Read the model definition and answer for the solid it produces. Units are mm, in the model's axes. Face numbers are marked on the shaded views. Give positions to 0.01 mm unless a question says otherwise; leave off trailing zeros. Write each loop counter-clockwise with the first axis right and the second up, starting at its lowest first coordinate (ties: lowest second). Pieces come first, ordered by that corner, then holes. Notation, with made-up numbers: M 22.25,-1 L 57.25,-1 A30 ccw 57.25,23 Z; hole C 33.25,35 d6. An arc over 180 degrees is marked long. Use a Markdown table: item, result. Add a question column.
Item 1: A cutting plane is placed at A-A on x = 55.5. Determine the outline of the cut face in (y, z), then the cut area to 3 significant figures.
Item 2: Given P1, Ø10, axis at x = 97.5, y = -38.5, coming from the +Z side; P2, Ø3, axis at x = 80.5, z = -8, coming from the +Y side; P3, Ø3, axis at x = 27, z = -3.5, coming from the -Y side; P4, Ø4, axis at y = -60, z = -7.5, coming from the +X side, each flat-ended and moving along its own axis, determine where each tip first touches the part or whether it passes through.
Item 3: A cutting plane is placed at C-C on z = -8. Count the separate pieces of the cut face and the enclosed holes in it, then the cut area to 3 significant figures.
Item 4: Consider probe 1 along Y at (x, z) = (114, -10.5); probe 2 along X at (y, z) = (-56.5, -9.25); probe 3 along X at (y, z) = (27.5, -4.75). Determine where each line is inside the solid, lowest interval first. Write a range as [from, to].
Item 5: A cutting plane is placed at B-B on y = -19. Determine the outline of the cut face in (x, z), then the cut area to 3 significant figures.
Item 6: The mould has two halves that part along Y. Classify the marked faces 1 and 2: pulls with the +Y half, pulls with the -Y half, needs draft (parallel to the pull), parting line crosses it, or undercut.
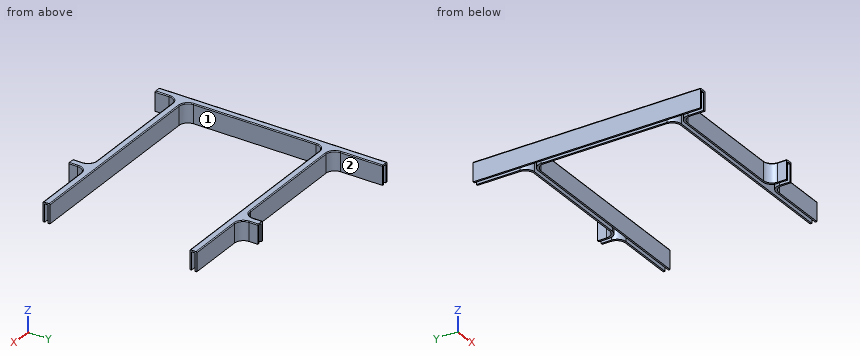
from build123d import *

# Parameters (mm, degrees)
F0_W     = 2
F0_H     = 10
F0_H_2   = 1
F1_DEPTH = 0.9
F0_W_2   = 1
F0_H_3   = 130
F0_W_3   = 76
F0_W_4   = 38
F2_DEPTH = 11
F3_R     = 5
F4_R     = 0.5


with BuildPart() as f1:
    # F0 (on Top) → F1 (new body)
    with BuildSketch(Plane.XY):
        Polygon((-1, -65), (1, -65), (1, -51), (1, -49), (1, 33), (1, 35), (1, 65), (-1, 65), align=None)
        Polygon((1, 35), (1, 33), (2, 33), (79, 33), (81, 33), (120, 33), (120, 35), (82, 35), (81, 35), (79, 35), (78, 35), (2, 35), align=None)
        with Locations((80, 41)):
            Rectangle(F0_W, F0_H)
        with Locations((80, 35.5)):
            Rectangle(F0_W, F0_H_2)
        Polygon((1, -49), (1, -51), (2, -51), (78, -51), (79, -51), (81, -51), (82, -51), (120, -51), (120, -49), (81, -49), (79, -49), (2, -49), align=None)
        with Locations((80, -57)):
            Rectangle(F0_W, F0_H)
        with Locations((80, -51.5)):
            Rectangle(F0_W, F0_H_2)
    extrude(amount=-F1_DEPTH)

    # F0 (on Top) → F2 (join)
    with BuildSketch(Plane.XY):
        Polygon((1, -51), (1, -65), (2, -65), (2, -52), (2, -51), align=None)
        with Locations((-1.5, 0)):
            Rectangle(F0_W_2, F0_H_3)
        Polygon((1, 33), (1, -49), (2, -49), (2, -48), (2, 32), (2, 33), align=None)
        with Locations((40, -51.5)):
            Rectangle(F0_W_3, F0_H_2)
        Polygon((2, 65), (1, 65), (1, 35), (2, 35), (2, 36), align=None)
        Polygon((2, -48), (2, -49), (79, -49), (79, -48), (78, -48), align=None)
        with Locations((78.5, -51.5)):
            Rectangle(F0_W_2, F0_H_2)
        with Locations((78.5, -57)):
            Rectangle(F0_W_2, F0_H)
        Polygon((79, 33), (2, 33), (2, 32), (78, 32), (79, 32), align=None)
        with Locations((80, -48.5)):
            Rectangle(F0_W, F0_H_2)
        with Locations((40, 35.5)):
            Rectangle(F0_W_3, F0_H_2)
        with Locations((80, 32.5)):
            Rectangle(F0_W, F0_H_2)
        Polygon((81, -48), (81, -49), (120, -49), (120, -48), (82, -48), align=None)
        with Locations((81.5, -51.5)):
            Rectangle(F0_W_2, F0_H_2)
        with Locations((81.5, -57)):
            Rectangle(F0_W_2, F0_H)
        with Locations((78.5, 35.5)):
            Rectangle(F0_W_2, F0_H_2)
        with Locations((78.5, 41)):
            Rectangle(F0_W_2, F0_H)
        Polygon((120, 33), (81, 33), (81, 32), (82, 32), (120, 32), align=None)
        with Locations((101, -51.5)):
            Rectangle(F0_W_4, F0_H_2)
        with Locations((81.5, 35.5)):
            Rectangle(F0_W_2, F0_H_2)
        with Locations((81.5, 41)):
            Rectangle(F0_W_2, F0_H)
        with Locations((101, 35.5)):
            Rectangle(F0_W_4, F0_H_2)
    extrude(amount=-F2_DEPTH)

    # F3
    f3_edges = [f1.edges().sort_by_distance(p)[0] for p in [
        (78, -52, -5.5),
        (81, -51, -5.95),
        (82, -52, -5.5),
        (79, -51, -5.95),
        (1, -49, -5.95),
        (1, -51, -5.95),
        (2, -52, -5.5),
        (2, -48, -5.5),
        (2, 36, -5.5),
        (1, 33, -5.95),
        (1, 35, -5.95),
        (2, 32, -5.5),
        (81, 35, -5.95),
        (79, 35, -5.95),
        (82, 36, -5.5),
        (78, 36, -5.5),
    ]]
    fillet(f3_edges, radius=F3_R)

    # F4
    f4_edges = [f1.edges().sort_by_distance(p)[0] for p in [
        (63.5, 32, 0),
        (103.5, 36, 0),
        (82, 43.5, 0),
        (78, 43.5, 0),
        (40, 36, 0),
        (2, 53, 0),
        (40, -52, 0),
        (103.5, -52, 0),
        (-2, 0, 0),
        (2, -61, 0),
        (3.464466, -53.464466, 0),
        (76.535534, -53.464466, 0),
        (78, -59.5, 0),
        (3.464466, 37.464466, 0),
        (82, -59.5, 0),
        (83.464466, -53.464466, 0),
        (76.535534, 37.464466, 0),
        (63.5, -48, 0),
        (3.464466, -46.535534, 0),
        (83.464466, 37.464466, 0),
        (2, -8, 0),
        (3.464466, 30.535534, 0),
    ]]
    fillet(f4_edges, radius=F4_R)


solid = f1.part
Filled in:
| question | item | result |
|---|---|---|
| 1 | outline | M -52,-11 L -51,-11 L -51,-0.9 L -49,-0.9 L -49,-11 L -48,-11 L -48,-0.5 A0.5 ccw -48.5,0 L -51.5,0 A0.5 ccw -52,-0.5 Z; M 32,-11 L 33,-11 L 33,-0.9 L 35,-0.9 L 35,-11 L 36,-11 L 36,-0.5 A0.5 ccw 35.5,0 L 32.5,0 A0.5 ccw 32,-0.5 Z |
| 1 | area | 47.4 mm² |
| 2 | P1 | through |
| 2 | P2 | y = 46 |
| 2 | P3 | y = -52 |
| 2 | P4 | x = 82 |
| 3 | separate pieces | 6 |
| 3 | enclosed holes | 0 |
| 3 | area | 764 mm² |
| 4 | probe 1 | [-52, -51], [-49, -48], [32, 33], [35, 36] |
| 4 | probe 2 | [-2, -1], [1, 2.03], [77.97, 79], [81, 82.03] |
| 4 | probe 3 | [-2, -1], [1, 2.03] |
| 5 | outline | M -2,-11 L -1,-11 L -1,-0.9 L 1,-0.9 L 1,-11 L 2,-11 L 2,-0.5 A0.5 ccw 1.5,0 L -1.5,0 A0.5 ccw -2,-0.5 Z |
| 5 | area | 23.7 mm² |
| 6 | face 1 | undercut |
| 6 | face 2 | needs draft |
